For this review, take the finished solid that the model builds, in its own axes (mm). Give positions to 0.01 mm unless a question says otherwise; leave off trailing zeros. Order: outer loops, then holes, each group sorted by start corner. A loop starts at its lowest first (then second) coordinate and runs counter-clockwise, first axis right, second up. Notation, with made-up numbers: M -39,42 L -10,42 A16 cw -10,72 Z; hole C 54,62 d2. An arc over 180 degrees is marked long. Use CSV: the item, a comma, the result in double quotes. Start each with the question number.
(1) Consider section A-A (x = 16). Write out the cut boundary in (y, z).
(2) Clearance check with flat-ended pins moving along their axes: P1, Ø3, axis at x = 7.5, y = -56, coming from the +Z side; P2, Ø8, axis at y = -58.5, z = 75.5, coming from the -X side; P3, Ø6, axis at x = -14, y = -67.5, coming from the -Z side. State where each tip first meets the part, or that it passes through.
(3) Wall thickness on L1, parallel to X at y = -164, z = 73.75; L2, parallel to Z at x = 59, y = -25; L3, parallel to Z at x = 74.5, y = -77: over which ranges is each line inside the solid? List them lowest first. Write a range as from..to.
(4) Consider section B-B (y = -131.5). Write out the cut boundary in (x, z).
(5) Draft analysis for pull direction X (two halves, no side actions). For faces 1 (the face through (100.957, -134, 72)), 2 (the face through (103.957, -135, 67)), 3 (the face through (2.557, 17.252, 59.827)), state which applies: pulls with the +X half, pulls with the -X half, needs draft (parallel to the pull), parting line crosses it, or undercut.
```python
from build123d import *

# Parameters (mm, degrees)
BOSS_EXTRUDE1_DEPTH      = 5
BOSS_EXTRUDE1_DEPTH_BACK = 5
SKETCH2_W                = 200
SKETCH2_H                = 300
SKETCH4_W                = 194
SKETCH4_H                = 294
CUT_EXTRUDE1_DEPTH       = 1


with BuildPart() as part:
    # Sketch2 → Boss-Extrude1 (new, two sides: drawn at the far end of the back side and taken through both)
    with BuildSketch(Plane(origin=(0, 3.030412593, 60.608251865), x_dir=(1, 0, 0), z_dir=(0, 0.0499376169438969, 0.9987523388778444)).offset(-BOSS_EXTRUDE1_DEPTH_BACK)):
        with Locations((3.957252563, -135.75687777)):
            Rectangle(SKETCH2_W, SKETCH2_H)
    extrude(amount=BOSS_EXTRUDE1_DEPTH + BOSS_EXTRUDE1_DEPTH_BACK)

    # Sketch4 → Cut-Extrude1 (cut)
    with BuildSketch(Plane(origin=(0, 3.280100678, 65.60201356), x_dir=(1, 0, 0), z_dir=(0, 0.049937616943896895, 0.9987523388778444))):
        with Locations((3.957252563, -135.75687777)):
            Rectangle(SKETCH4_W, SKETCH4_H)
    extrude(amount=-CUT_EXTRUDE1_DEPTH, mode=Mode.SUBTRACT)


solid = part.part
```
Check result:
1,outline,"M -282.62,69.88 L 17.01,54.9 L 17.51,64.89 L 14.51,65.04 L 14.46,64.04 L -279.17,78.72 L -279.12,79.72 L -282.12,79.87 Z"
2,P1,"stops at z = 67.64"
2,P2,"passes through"
2,P3,"stops at z = 58.98"
3,L1,"x = -96.04..-93.04, 100.96..103.96"
3,L2,"z = 57..66.01"
3,L3,"z = 59.6..68.61"
4,outline,"M -96.04,62.33 L 103.96,62.33 L 103.96,72.34 L 100.96,72.34 L 100.96,71.34 L -93.04,71.34 L -93.04,72.34 L -96.04,72.34 Z"
5,face 1,"undercut"
5,face 2,"pulls with the +X half"
5,face 3,"needs draft"
